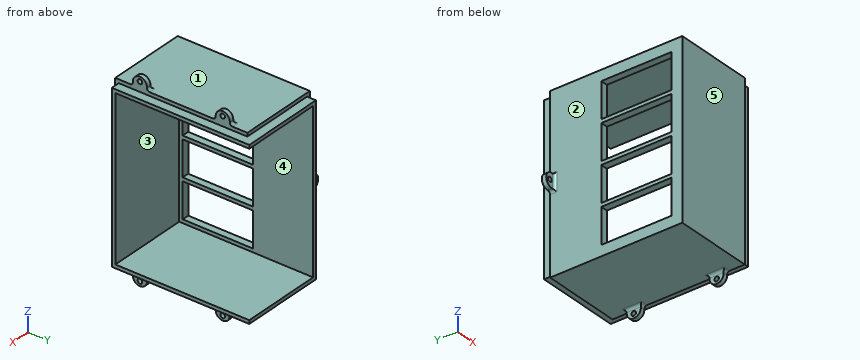
```python
from build123d import *

# Parameters (mm, degrees)
SKETCH1_W           = 50
SKETCH1_H           = 98
BOSS_EXTRUDE3_DEPTH = 80
SKETCH4_W           = 90
SKETCH4_H           = 76
CUT_EXTRUDE2_DEPTH  = 46
SKETCH6_W           = 48
SKETCH6_H           = 2
CUT_EXTRUDE3_DEPTH  = 5
SKETCH7_W           = 2
SKETCH7_H           = 73
CUT_EXTRUDE4_DEPTH  = 5
SKETCH10_R          = 1.3
BOSS_EXTRUDE6_DEPTH = 2.5
FILLET2_R           = 1.5
FILLET3_R           = 1.5
SKETCH12_R          = 1.3
BOSS_EXTRUDE7_DEPTH = 2.5
FILLET4_R           = 1.5
CUT_EXTRUDE5_REACH  = 52
SKETCH14_W          = 20
SKETCH14_H          = 40


with BuildPart() as part:
    # Sketch1 → Boss-Extrude3 (new body)
    with BuildSketch(Plane(origin=(0, 0, 0), x_dir=(1, 0, 0), z_dir=(0, 1, 0))):
        Rectangle(SKETCH1_W, SKETCH1_H)
    extrude(amount=BOSS_EXTRUDE3_DEPTH)

    # Sketch4 → Cut-Extrude2 (cut)
    with BuildSketch(Plane(origin=(25, 0, 0), x_dir=(0, 0, -1), z_dir=(1, 0, 0))):
        with Locations((0, 42)):
            Rectangle(SKETCH4_W, SKETCH4_H)
    extrude(amount=-CUT_EXTRUDE2_DEPTH, mode=Mode.SUBTRACT)

    # Sketch6 → Cut-Extrude3 (cut)
    with BuildSketch(Plane(origin=(0, 80, 0), x_dir=(1, 0, 0), z_dir=(0, 1, 0))):
        with Locations((1, 48)):
            Rectangle(SKETCH6_W, SKETCH6_H)
        Polygon((-25, 49), (-25, -47), (-23, -47), (-23, 47), (-23, 49), align=None)
        Polygon((-25, -49), (25, -49), (25, -47), (-23, -47), (-25, -47), align=None)
    extrude(amount=-CUT_EXTRUDE3_DEPTH, mode=Mode.SUBTRACT)

    # Sketch7 → Cut-Extrude4 (cut)
    with BuildSketch(Plane(origin=(25, 0, 0), x_dir=(0, 0, -1), z_dir=(1, 0, 0))):
        Polygon((-47, 75), (-49, 75), (-49, 0), (-47, 0), (-47, 2), align=None)
        Polygon((47, 2), (-47, 2), (-47, 0), (49, 0), (49, 2), align=None)
        with Locations((48, 38.5)):
            Rectangle(SKETCH7_W, SKETCH7_H)
    extrude(amount=-CUT_EXTRUDE4_DEPTH, mode=Mode.SUBTRACT)

    # Sketch10 → Boss-Extrude6 (add)
    with BuildSketch(Plane(origin=(20, 0, 0), x_dir=(0, 0, -1), z_dir=(1, 0, 0))):
        with BuildLine():
            Line((-49, 10), (-51, 10))
            ThreePointArc((-51, 10), (-55, 14), (-51, 18))
            Line((-51, 18), (-49, 18))
            Line((-49, 18), (-49, 10))
        make_face()
        with Locations((-52.4, 14)):
            Circle(SKETCH10_R, mode=Mode.SUBTRACT)
        with BuildLine():
            Line((-49, 65), (-49, 57))
            Line((-49, 57), (-51, 57))
            ThreePointArc((-51, 57), (-55, 61), (-51, 65))
            Line((-51, 65), (-49, 65))
        make_face()
        with Locations((-52.4, 61)):
            Circle(SKETCH10_R, mode=Mode.SUBTRACT)
        with BuildLine():
            Line((49, 10), (49, 18))
            Line((49, 18), (51, 18))
            ThreePointArc((51, 18), (55, 14), (51, 10))
            Line((51, 10), (49, 10))
        make_face()
        with Locations((52.4, 14)):
            Circle(SKETCH10_R, mode=Mode.SUBTRACT)
        with BuildLine():
            Line((49, 65), (51, 65))
            ThreePointArc((51, 65), (55, 61), (51, 57))
            Line((51, 57), (49, 57))
            Line((49, 57), (49, 65))
        make_face()
        with Locations((52.4, 61)):
            Circle(SKETCH10_R, mode=Mode.SUBTRACT)
    extrude(amount=-BOSS_EXTRUDE6_DEPTH)

    # Fillet2
    fillet2_edges = [part.edges().sort_by_distance(p)[0] for p in [
        (17.5, 61, 49),
        (18.75, 65, 49),
        (18.75, 57, 49),
        (17.5, 14, 49),
        (18.75, 18, 49),
        (18.75, 10, 49),
    ]]
    fillet(fillet2_edges, radius=FILLET2_R)

    # Fillet3
    fillet3_edges = [part.edges().sort_by_distance(p)[0] for p in [
        (17.5, 14, -49),
        (18.75, 10, -49),
        (18.75, 18, -49),
        (17.5, 61, -49),
        (18.75, 57, -49),
        (18.75, 65, -49),
    ]]
    fillet(fillet3_edges, radius=FILLET3_R)

    # Sketch12 → Boss-Extrude7 (add)
    with BuildSketch(Plane(origin=(0, 75, 0), x_dir=(1, 0, 0), z_dir=(0, 1, 0))):
        with BuildLine():
            Line((-25, 4), (-27, 4))
            ThreePointArc((-27, 4), (-31, 0), (-27, -4))
            Line((-27, -4), (-25, -4))
            Line((-25, -4), (-25, 4))
        make_face()
        with Locations((-28.4, 0)):
            Circle(SKETCH12_R, mode=Mode.SUBTRACT)
    extrude(amount=-BOSS_EXTRUDE7_DEPTH)

    # Fillet4
    fillet4_edges = [part.edges().sort_by_distance(p)[0] for p in [
        (-25, 72.5, 0),
        (-25, 73.75, -4),
        (-25, 73.75, 4),
    ]]
    fillet(fillet4_edges, radius=FILLET4_R)

    # Sketch14 → Cut-Extrude5 (cut, up to next)
    with BuildSketch(Plane.ZY.offset(25), mode=Mode.PRIVATE) as cut_extrude5_sk1:
        with Locations((33, 26)):
            Rectangle(SKETCH14_W, SKETCH14_H)
    cut_extrude5_tool1 = extrude(cut_extrude5_sk1.sketch, amount=-CUT_EXTRUDE5_REACH, mode=Mode.PRIVATE) & part.part
    add(cut_extrude5_tool1.solids().sort_by_distance((-25, 26, 33))[0], mode=Mode.SUBTRACT)
    # Sketch14 → Cut-Extrude5 (cut, up to next)
    with BuildSketch(Plane.ZY.offset(25), mode=Mode.PRIVATE) as cut_extrude5_sk2:
        with Locations((11, 26)):
            Rectangle(SKETCH14_W, SKETCH14_H)
    cut_extrude5_tool2 = extrude(cut_extrude5_sk2.sketch, amount=-CUT_EXTRUDE5_REACH, mode=Mode.PRIVATE) & part.part
    add(cut_extrude5_tool2.solids().sort_by_distance((-25, 26, 11))[0], mode=Mode.SUBTRACT)
    # Sketch14 → Cut-Extrude5 (cut, up to next)
    with BuildSketch(Plane.ZY.offset(25), mode=Mode.PRIVATE) as cut_extrude5_sk3:
        with Locations((-11, 26)):
            Rectangle(SKETCH14_W, SKETCH14_H)
    cut_extrude5_tool3 = extrude(cut_extrude5_sk3.sketch, amount=-CUT_EXTRUDE5_REACH, mode=Mode.PRIVATE) & part.part
    add(cut_extrude5_tool3.solids().sort_by_distance((-25, 26, -11))[0], mode=Mode.SUBTRACT)
    # Sketch14 → Cut-Extrude5 (cut, up to next)
    with BuildSketch(Plane.ZY.offset(25), mode=Mode.PRIVATE) as cut_extrude5_sk4:
        with Locations((-33, 26)):
            Rectangle(SKETCH14_W, SKETCH14_H)
    cut_extrude5_tool4 = extrude(cut_extrude5_sk4.sketch, amount=-CUT_EXTRUDE5_REACH, mode=Mode.PRIVATE) & part.part
    add(cut_extrude5_tool4.solids().sort_by_distance((-25, 26, -33))[0], mode=Mode.SUBTRACT)


solid = part.part
```
Could you check a few things on this model? Use its own coordinates, in mm. Face numbers are marked on the shaded views. A direction names the side the tool comes from. Round coordinates to 2 decimals unless told otherwise and drop trailing zeros. Loops run counter-clockwise (first coordinate to the right, second up) from the corner with the lowest first, then second, coordinate; pieces in that order, holes last.
Q1. On a 3-axis mill with a long thin cutter (end or side, diameter ignored), from which of +Z, -Z, +X, -X, +Y, -Y can I reach the whole of each face in a straight line? I mean the marked faces 4 and 5. Say none if no direction works.
Q2. I want a section at D-D (x = -18). Write out the boundary of the cut face in (y, z), and give its area (3 significant figures).
Q3. I want a section at C-C (x = -28.4). Write out the boundary of the cut face in (y, z).
Q4. Thinking about a two-plate mould opening in Z: for the marked faces 1, 2 and 3, which applies, pulls with the +Z half, pulls with the -Z half, needs draft (parallel to the pull), parting line crosses it, or undercut?
Q5. Please list where these lines run through material, in increasing order: L1, parallel to Z at x = 15.5, y = 5; L2, parallel to X at y = 74.25, z = 0; L3, parallel to Y at x = 18.4, z = 52.4.
Q6. For P1, Ø14, axis at x = 4.5, y = 27, coming from the -Z side; P2, Ø12, axis at x = -23.5, y = 49, coming from the +Z side; P3, Ø2, axis at y = 15, z = 52, coming from the -X side, each with a flat end and sliding along its axis, tell me the tip position at first contact or that it passes through.
Q7. I want a section at B-B (y = 40.5). Write out the boundary of the cut face in (x, z), and give its area (3 significant figures).
Q8. I want a section at A-A (z = 40). Write out the boundary of the cut face in (x, y).
Answer below:
1. face 4: +X, +Y
1. face 5: +Z, -Z, +X, -X, -Y
2. outline: (0, -49) - (75, -49) - (75, -47) - (80, -47) - (80, -45) - (4, -45) - (4, 45) - (80, 45) - (80, 47) - (75, 47) - (75, 49) - (0, 49) - close
2. area: 980 mm2
3. outline: (72.5, -3.75) - (75, -3.75) - (75, -1.3) - (72.5, -1.3) - close; (72.5, 1.3) - (75, 1.3) - (75, 3.75) - (72.5, 3.75) - close
4. face 1: pulls with the +Z half
4. face 2: needs draft
4. face 3: undercut
5. L1: z = -49 to -45, 45 to 49
5. L2: x = -31 to -29.7, -27.1 to -21
5. L3: y = 10.25 to 12.7, 15.3 to 17.75, 57.25 to 59.7, 62.3 to 64.75
6. P1: stops at z = -49
6. P2: stops at z = 49
6. P3: stops at x = 17.5
7. outline: (-25, -49) - (20, -49) - (20, -47) - (25, -47) - (25, -45) - (-21, -45) - (-21, -43) - (-25, -43) - close; (-25, -23) - (-21, -23) - (-21, -21) - (-25, -21) - close; (-25, -1) - (-21, -1) - (-21, 1) - (-25, 1) - close; (-25, 21) - (-21, 21) - (-21, 23) - (-25, 23) - close; (-25, 43) - (-21, 43) - (-21, 45) - (25, 45) - (25, 47) - (20, 47) - (20, 49) - (-25, 49) - close
7. area: 420 mm2
8. outline: (-25, 0) - (20, 0) - (20, 2) - (25, 2) - (25, 4) - (-21, 4) - (-21, 6) - (-25, 6) - close; (-25, 46) - (-21, 46) - (-21, 80) - (-23, 80) - (-23, 75) - (-25, 75) - close
